from build123d import *

# Parameters (mm, degrees)
BASE_FLANGE1_DEPTH      = 242
EXTRUDE_THIN1_DEPTH     = 2
CUT_EXTRUDE3_DEPTH      = 1473.940690723
CUT_EXTRUDE3_DEPTH_BACK = 1473.940690723


# Read off the part's stored shape, not the designer's step: Base-Flange1
with BuildPart() as part:
    # Base-Flange1 outline → Base-Flange1 (new body)
    with BuildSketch(Plane.XY):
        with BuildLine():
            Line((871.769127642, 521.057153497), (905.269127642, 521.057153497))
            Line((905.269127642, 521.057153497), (905.269127642, 523.557153497))
            Line((905.269127642, 523.557153497), (871.769127642, 523.557153497))
            ThreePointArc((871.769127642, 523.557153497), (868.940700517, 524.728726372), (867.769127642, 527.557153497))
            Line((867.769127642, 527.557153497), (867.769127642, 756.805124112))
            ThreePointArc((867.769127642, 756.805124112), (867.77210353, 756.959390926), (867.781026767, 757.1134282))
            ThreePointArc((867.781026767, 757.1134282), (784.657582784, 1012.417540201), (545.544536696, 1134.54308108))
            ThreePointArc((545.544536696, 1134.54308108), (545.498432474, 1134.547059372), (545.45237736, 1134.551570763))
            ThreePointArc((545.45237736, 1134.551570763), (231.971479061, 1042.712636382), (72.799654121, 757.46012787))
            ThreePointArc((72.799654121, 757.46012787), (72.781664067, 757.29368801), (72.76796633, 757.126840052))
            ThreePointArc((72.76796633, 757.126840052), (196.842388714, 389.59572995), (545.115755529, 218.776406833))
            ThreePointArc((545.115755529, 218.776406833), (725.093462287, 208.692500871), (905.169857989, 200.559125168))
            Line((905.169857989, 200.559125168), (905.269127642, 203.057153497))
            ThreePointArc((905.269127642, 203.057153497), (725.219790585, 211.189307063), (545.269127642, 221.271697797))
            ThreePointArc((545.269127642, 221.271697797), (198.721595151, 391.244542603), (75.262011332, 756.954388532))
            ThreePointArc((75.262011332, 756.954388532), (75.270440709, 757.057064199), (75.281511511, 757.159488728))
            ThreePointArc((75.281511511, 757.159488728), (233.530616685, 1040.758387199), (545.194264845, 1132.064930876))
            ThreePointArc((545.194264845, 1132.064930876), (545.269104404, 1132.057599865), (545.344023766, 1132.051135141))
            ThreePointArc((545.344023766, 1132.051135141), (782.756272141, 1010.794266398), (865.28846372, 757.306118255))
            ThreePointArc((865.28846372, 757.306118255), (865.27396346, 757.055807685), (865.269127642, 756.805124112))
            Line((865.269127642, 756.805124112), (865.269127642, 527.557153497))
            ThreePointArc((865.269127642, 527.557153497), (867.172933564, 522.960959419), (871.769127642, 521.057153497))
        make_face()
    extrude(amount=BASE_FLANGE1_DEPTH)

    # Sketch9 → Extrude-Thin1 (add)
    with BuildSketch(Plane.XY):
        with BuildLine():
            Line((905.269127642, 203.057153497), (905.269127642, 521.057153497))
            Line((905.269127642, 521.057153497), (865.269127642, 521.057153497))
            Line((865.269127642, 521.057153497), (865.269127642, 757.057153497))
            ThreePointArc((865.269127642, 757.057153497), (782.812941082, 1010.7278743), (545.269127642, 1132.057153497))
            ThreePointArc((545.269127642, 1132.057153497), (233.519744905, 1040.749713195), (75.269127642, 757.057153497))
            ThreePointArc((75.269127642, 757.057153497), (198.687627947, 391.283260157), (545.269127642, 221.271697797))
            ThreePointArc((545.269127642, 221.271697797), (725.219790584, 211.189307063), (905.269127642, 203.057153497))
        make_face()
        with BuildLine():
            Line((895.269127642, 213.465697296), (895.269127642, 511.057153497))
            Line((895.269127642, 511.057153497), (855.269127642, 511.057153497))
            Line((855.269127642, 511.057153497), (855.269127642, 757.449526591))
            ThreePointArc((855.269127642, 757.449526591), (775.293432889, 1004.134267456), (544.352108556, 1122.098574947))
            ThreePointArc((544.352108556, 1122.098574947), (239.902349284, 1033.049195687), (85.227547592, 756.110297031))
            ThreePointArc((85.227547592, 756.110297031), (206.289423946, 397.781672568), (545.882616091, 231.252861653))
            ThreePointArc((545.882616091, 231.252861653), (720.529084068, 221.440244534), (895.269127642, 213.465697296))
        make_face(mode=Mode.SUBTRACT)
    extrude(amount=EXTRUDE_THIN1_DEPTH)

    # Sketch11 → Cut-Extrude3 (cut, two sides: drawn at the far end of the back side and taken through both)
    with BuildSketch(Plane.XY.offset(2).offset(-CUT_EXTRUDE3_DEPTH_BACK)):
        Polygon((905.269127642, 521.057153497), (895.269127642, 521.057153497), (855.269127642, 521.057153497), (855.269127642, 511.057153497), (895.269127642, 511.057153497), (895.269127642, 213.465697296), (905.269127642, 213.465697296), align=None)
    extrude(amount=CUT_EXTRUDE3_DEPTH + CUT_EXTRUDE3_DEPTH_BACK, mode=Mode.SUBTRACT)


solid = part.part
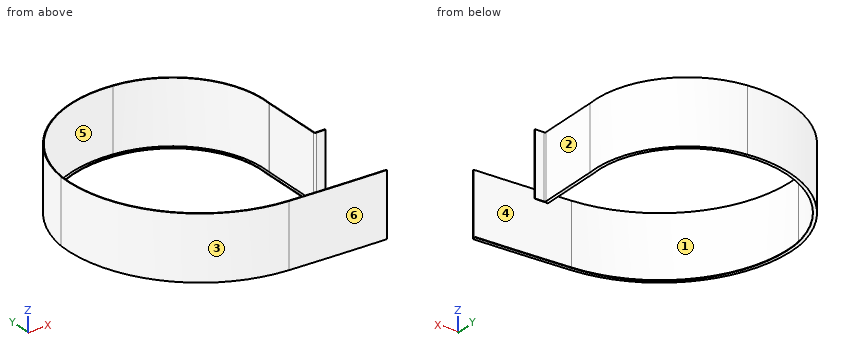
Geometry check sheet. Reference: the model listing, model coordinates, mm. Face numbers are marked on the shaded views. A direction names the side the tool comes from. Round coordinates to 2 decimals unless told otherwise and drop trailing zeros. Order: outer loops, then holes, each group sorted by start corner. A loop starts at its lowest first (then second) coordinate and runs counter-clockwise, first axis right, second up. Notation, with made-up numbers: (62.5, -25.75) -> (106.5, -25.75) arc R12 ccw to (106.5, -17.75) -> close; hole circle Ø10 at (-27, 29). An arc over 180 degrees is marked (long way). Use one line per item in the form item = value.
1. Set-up check for the marked faces 4, 5 and 6: record each of +Z, -Z, +X, -X, +Y, -Y from which the full face is reachable in a straight line by a thin tool's end or side.
Working result:
face_4 = +Z, +X
face_5 = +Z
face_6 = +Z, -Z, -X, -Y
2. Cross-section at B-B, the plane y = 675. Enter the section's corners in (x, z).
Working result:
outline = (73.79, 0) -> (86.35, 0) -> (86.35, 2) -> (76.3, 2) -> (76.3, 242) -> (73.79, 242) -> close; (855.27, 0) -> (867.77, 0) -> (867.77, 242) -> (865.27, 242) -> (865.27, 2) -> (855.27, 2) -> close
3. Scan lines: line 1 along Y through (x, z) = (721.5, 200); line 2 along Y through (x, z) = (835.5, 105); line 3 along X through (y, z) = (980.5, 138.5) (3 decimals). Record each from-to range of solid material in increasing order. Write a range as from..to.
Working result:
line_1 = 208.87..211.38, 1067.23..1070.31
line_2 = 203.47..205.98, 927.61..933.59
line_3 = 168.644..171.895, 805.884..808.903
4. Cross-section at C-C, the plane z = 182. Enter the section's corners in (x, y).
Working result:
outline = (72.77, 757.13) arc R504.5 ccw to (545.12, 218.78) arc R16637.6 ccw to (905.17, 200.56) -> (905.27, 203.06) arc R16635.1 cw to (545.27, 221.27) arc R502 cw to (75.26, 756.95) arc R4 cw to (75.28, 757.16) arc R428.76 cw to (545.19, 1132.06) arc R6.5 ccw to (545.34, 1132.05) arc R348.97 cw to (865.29, 757.31) arc R6.5 ccw to (865.27, 756.81) -> (865.27, 527.56) arc R6.5 ccw to (871.77, 521.06) -> (905.27, 521.06) -> (905.27, 523.56) -> (871.77, 523.56) arc R4 cw to (867.77, 527.56) -> (867.77, 756.81) arc R4 cw to (867.78, 757.11) arc R351.47 ccw to (545.54, 1134.54) arc R4 cw to (545.45, 1134.55) arc R431.26 ccw to (72.8, 757.46) arc R6.5 ccw to start
5. Go/stop test with flat-tipped pins: pin 1 (3 mm diameter, centred on x = 466.5, z = 183.5, fed in from -Y); pin 2 (2 mm diameter, centred on x = 448.5, z = 149, fed in from -Y); pin 3 (2 mm diameter, centred on x = 270, z = 161, fed in from +Y). Record where each tip stops, or that it passes through.
Working result:
pin_1 = 229.54
pin_2 = 233.96
pin_3 = 1070.45
6. Mould release check, pull along X, two halves, no side actions. Record for the marked faces 1, 2 and 3: pulls with the +X half, pulls with the -X half, needs draft (parallel to the pull), parting line crosses it, or undercut.
Working result:
face_1 = undercut
face_2 = pulls with the +X half
face_3 = pulls with the -X half
